For this review, take the finished solid that the model builds, in its own axes (mm). Round coordinates to 2 decimals unless told otherwise and drop trailing zeros. Write each loop counter-clockwise with the first axis right and the second up, starting at its lowest first coordinate (ties: lowest second). Pieces come first, ordered by that corner, then holes. Notation, with made-up numbers: (-29, 87) -> (24, 87) arc R38 cw to (24, 125) -> close; hole circle Ø1 at (-23.5, 6.25). An arc over 180 degrees is marked (long way). Answer as CSV lines item,"result". Start each with the question number.
Item 1: Wall thickness on probe 1 along Y at (x, z) = (74.5, 3.4); probe 2 along Y at (x, z) = (0, 2.55); probe 3 along Y at (x, z) = (79.5, 1.7): over which ranges is each line inside the solid? List them lowest first. Write a range as from..to.
Item 2: Take a section at A-A on y = 0. Give the boundary of the cut face in (x, z).
Item 3: Take a section at C-C on x = 75. Give the boundary of the cut face in (y, z), then the cut area to 3 significant figures.
Item 4: For pin 1 Ø3 at (x, y) = (-16.24, 9.38) entering from -Z, flat-tipped, find the tip position at first contact; note if it passes through.
Item 5: Take a section at B-B on y = -30. Give the boundary of the cut face in (x, z).
Item 6: Take a section at D-D on z = 3.1. Count the separate pieces of the cut face and the enclosed holes in it, then the cut area to 3 significant figures.
Item 7: Mouldability with a two-part tool opening along Y and no side actions: class faces 1 (the flat face through (95, -1, 2)), 2 (the flat face through (-1, 60, 2)), 3 (the cylindrical face through (17.313, 11.061, 2.465)), 4 (the cylindrical face through (-14.33, 9.98, 2.46)) as +Y half, -Y half, draft (parallel to the pull), parting line (faces both ways), or undercut.
```python
from build123d import *

# Parameters (mm, degrees)
SKETCH1_W           = 190
SKETCH1_H           = 120
SKETCH1_R           = 6
SKETCH1_R_2         = 15.25
SKETCH1_R_3         = 2
BOSS_EXTRUDE1_DEPTH = 5


with BuildPart() as part:
    # Sketch1 → Boss-Extrude1 (new body)
    with BuildSketch(Plane.XY):
        Rectangle(SKETCH1_W, SKETCH1_H)
        with Locations((-75, 30)):
            Circle(SKETCH1_R, mode=Mode.SUBTRACT)
        with Locations((75, 30)):
            Circle(SKETCH1_R, mode=Mode.SUBTRACT)
        with Locations((75, -30)):
            Circle(SKETCH1_R, mode=Mode.SUBTRACT)
        with Locations((-75, -30)):
            Circle(SKETCH1_R, mode=Mode.SUBTRACT)
        Circle(SKETCH1_R_2, mode=Mode.SUBTRACT)
        with Locations((0, 18.75)):
            Circle(SKETCH1_R_3, mode=Mode.SUBTRACT)
        with Locations((16.237976321, 9.375)):
            Circle(SKETCH1_R_3, mode=Mode.SUBTRACT)
        with Locations((16.237976321, -9.375)):
            Circle(SKETCH1_R_3, mode=Mode.SUBTRACT)
        with Locations((0, -18.75)):
            Circle(SKETCH1_R_3, mode=Mode.SUBTRACT)
        with Locations((-16.237976321, -9.375)):
            Circle(SKETCH1_R_3, mode=Mode.SUBTRACT)
        with Locations((-16.237976321, 9.375)):
            Circle(SKETCH1_R_3, mode=Mode.SUBTRACT)
    extrude(amount=BOSS_EXTRUDE1_DEPTH)


solid = part.part
```
Output values:
1,probe 1,"y = -60..-35.98, -24.02..24.02, 35.98..60"
1,probe 2,"y = -60..-20.75, -16.75..-15.25, 15.25..16.75, 20.75..60"
1,probe 3,"y = -60..-33.97, -26.03..26.03, 33.97..60"
2,outline,"(-95, 0) -> (-15.25, 0) -> (-15.25, 5) -> (-95, 5) -> close; (15.25, 0) -> (95, 0) -> (95, 5) -> (15.25, 5) -> close"
3,outline,"(-60, 0) -> (-36, 0) -> (-36, 5) -> (-60, 5) -> close; (-24, 0) -> (24, 0) -> (24, 5) -> (-24, 5) -> close; (36, 0) -> (60, 0) -> (60, 5) -> (36, 5) -> close"
3,area,"480 mm^2"
4,pin 1,"passes through"
5,outline,"(-95, 0) -> (-81, 0) -> (-81, 5) -> (-95, 5) -> close; (-69, 0) -> (69, 0) -> (69, 5) -> (-69, 5) -> close; (81, 0) -> (95, 0) -> (95, 5) -> (81, 5) -> close"
6,separate pieces,"1"
6,enclosed holes,"11"
6,area,"21,500 mm^2"
7,face 1,"draft"
7,face 2,"+Y half"
7,face 3,"undercut"
7,face 4,"undercut"
